Work out the finished part from the listing and answer in its coordinate system (mm). Face numbers are marked on the shaded views. A direction names the side the tool comes from. Coordinates: 2 decimals unless noted, no trailing zeros. Order: outer loops, then holes, each group sorted by start corner. A loop starts at its lowest first (then second) coordinate and runs counter-clockwise, first axis right, second up.
1. The part is cut by section A-A, the plane z = 4.2. Give the vertices of the cut face in (x, y), then the cut area to 3 significant figures.
2. A tool of negligible diameter and unlimited length cuts with its end or side. For the marked faces 1 and 2, from which of +Z, -Z, +X, -X, +Y, -Y can it reach the whole face along a straight path? Write none if from no direction.
3. Determine the mould class of the marked faces 3, 4 and 5 for opening direction X: +X half, -X half, draft (parallel to the pull), parting line (faces both ways), or undercut.
4. Flat-ended cylindrical pins translate along their axes: pin 1 Ø2.5 at (x, z) = (-5, 3.5) entering from +Y; pin 2 Ø3 at (x, z) = (-47, 4.5) entering from -Y. Find the tip coordinate at first contact, or state that the pin passes through.
5. Find the intervals of material crossed by probe 1 along X at (y, z) = (0.75, 2.35); probe 2 along Y at (x, z) = (0, 1.75); probe 3 along Y at (x, z) = (-20.75, 3.1), in increasing order.
6. The part is cut by section C-C, the plane y = 12.25. Give the vertices of the cut face in (x, z).
7. The part is cut by section B-B, the plane x = -4.5. Give the vertices of the cut face in (y, z).
```python
from build123d import *

# Parameters (mm, degrees)
SKETCH2_R           = 1.749985299
SKETCH2_R_2         = 1.75
BOSS_EXTRUDE1_DEPTH = 5
FILLET1_R           = 5


with BuildPart() as part:
    # Sketch2 → Boss-Extrude1 (new body)
    with BuildSketch(Plane.XY):
        with BuildLine():
            Line((-33.828383846, 0.147779708), (-21.999999142, -4.999968857))
            Line((-21.999999142, -4.999968857), (0, -4.999968857))
            ThreePointArc((0, -4.999968857), (4.999968857, 0), (0, 4.999968857))
            Line((0, 4.999968857), (-8.7, 4.999968857))
            ThreePointArc((-8.7, 4.999968857), (-11.628806388, 5.263812443), (-14.523326425, 5.782728669))
            Line((-14.523326425, 5.782728669), (-38.709257265, 12.859504023))
            ThreePointArc((-38.709257265, 12.859504023), (-48.20223144, 13.862553465), (-57.417402301, 11.371912412))
            Line((-57.417402301, 11.371912412), (-58.891567994, 7.653467104))
            Line((-58.891567994, 7.653467104), (-52.198366439, 4.999968857))
            ThreePointArc((-52.198366439, 4.999968857), (-42.578635596, 4.219761872), (-33.828383846, 0.147779708))
        make_face()
        Circle(SKETCH2_R, mode=Mode.SUBTRACT)
        with Locations((-20.75, 0)):
            Circle(SKETCH2_R_2, mode=Mode.SUBTRACT)
    extrude(amount=BOSS_EXTRUDE1_DEPTH)

    # Fillet1
    fillet1_edges = [part.edges().sort_by_distance(p)[0] for p in [
        (-21.999999142, -4.999968857, 2.5),
    ]]
    fillet(fillet1_edges, radius=FILLET1_R)


solid = part.part
```
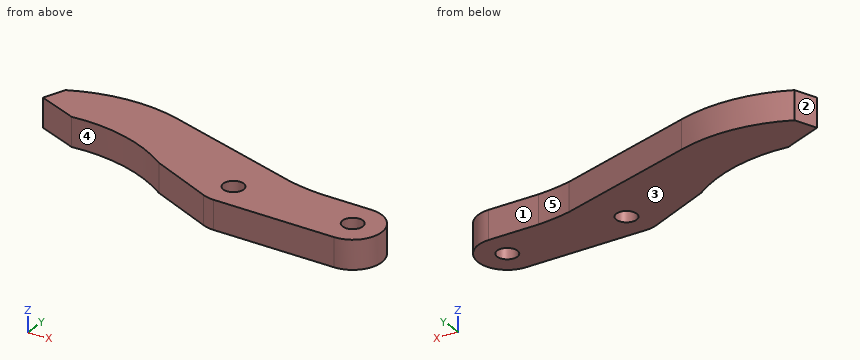
Geometry says:
1. outline: (-58.89, 7.65) - (-52.2, 5) arc R27.36 cw to (-33.83, 0.15) - (-22.95, -4.58) arc R5 ccw to (-20.96, -5) - (0, -5) arc R5 ccw to (0, 5) - (-8.7, 5) arc R33.6 cw to (-14.52, 5.78) - (-38.71, 12.86) arc R26 ccw to (-57.42, 11.37) - close; hole circle Ø3.5 at (-20.75, 0); hole circle Ø3.5 at (0, 0)
1. area: 610 mm2
2. face 1: +Z, -Z, +X, +Y
2. face 2: +Z, -Z, -X, +Y
3. face 3: draft
3. face 4: undercut
3. face 5: +X half
4. pin 1: stops at y = 5
4. pin 2: stops at y = 4.82
5. probe 1: x = -34.72 to -22.33, -19.17 to -1.58, 1.58 to 4.94
5. probe 2: y = -5 to -1.75, 1.75 to 5
5. probe 3: y = -5 to -1.75, 1.75 to 7.6
6. outline: (-55.37, 0) - (-36.63, 0) - (-36.63, 5) - (-55.37, 5) - close
7. outline: (-5, 0) - (5, 0) - (5, 5) - (-5, 5) - close
